from build123d import *

# Parameters (mm, degrees)
BOSS_EXTRUDE1_DEPTH = 6.35
BOSS_EXTRUDE2_DEPTH = 6.35
FILLET1_R           = 10
FILLET2_R           = 5
CUT_EXTRUDE1_DEPTH  = 7.35
SKETCH4_R           = 1.85
CUT_EXTRUDE2_DEPTH  = 7.35


with BuildPart() as part:
    # Sketch1 → Boss-Extrude1 (new body)
    with BuildSketch(Plane.XY):
        Polygon((-100, 0), (0, -100), (25.4, -100), (25.4, 25.4), (-100, 25.4), align=None)
    extrude(amount=BOSS_EXTRUDE1_DEPTH)

    # Sketch2 → Boss-Extrude2 (add)
    with BuildSketch(Plane.XY):
        Polygon((24.2, 37.7), (84.2, 37.7), (84.2, -22.3), (25.4, -100), (24.2, -22.3), (-100, 25.4), align=None)
    extrude(amount=BOSS_EXTRUDE2_DEPTH)

    # Fillet1
    fillet1_edges = [part.edges().sort_by_distance(p)[0] for p in [
        (84.2, 37.7, 3.175),
    ]]
    fillet(fillet1_edges, radius=FILLET1_R)

    # Fillet2
    fillet2_edges = [part.edges().sort_by_distance(p)[0] for p in [
        (84.2, -22.3, 3.175),
        (25.4, -100, 3.175),
        (0, -100, 3.175),
        (-100, 0, 3.175),
        (-100, 25.4, 3.175),
    ]]
    fillet(fillet2_edges, radius=FILLET2_R)

    # Sketch3 → Cut-Extrude1 (cut, through all)
    with BuildSketch(Plane.XY.offset(6.35)):
        with BuildLine():
            Line((43.7, 31.2), (64.7, 31.2))
            ThreePointArc((64.7, 31.2), (73.892388155, 27.392388155), (77.7, 18.2))
            Line((77.7, 18.2), (77.7, -2.8))
            ThreePointArc((77.7, -2.8), (73.892388155, -11.992388155), (64.7, -15.8))
            Line((64.7, -15.8), (43.7, -15.8))
            ThreePointArc((43.7, -15.8), (34.507611845, -11.992388155), (30.7, -2.8))
            Line((30.7, -2.8), (30.7, 18.2))
            ThreePointArc((30.7, 18.2), (34.507611845, 27.392388155), (43.7, 31.2))
        make_face()
    extrude(amount=-CUT_EXTRUDE1_DEPTH, mode=Mode.SUBTRACT)

    # Sketch4 → Cut-Extrude2 (cut, through all)
    with BuildSketch(Plane(origin=(0, 0, 0), x_dir=(-1, 0, 0), z_dir=(0, 0, -1))):
        with Locations((-77.581727984, 31.081727984)):
            Circle(SKETCH4_R)
        with Locations((-30.821727984, 31.081727984)):
            Circle(SKETCH4_R)
        with Locations((-30.821727984, -15.678272016)):
            Circle(SKETCH4_R)
        with Locations((-77.581727984, -15.678272016)):
            Circle(SKETCH4_R)
    extrude(amount=-CUT_EXTRUDE2_DEPTH, mode=Mode.SUBTRACT)


solid = part.part
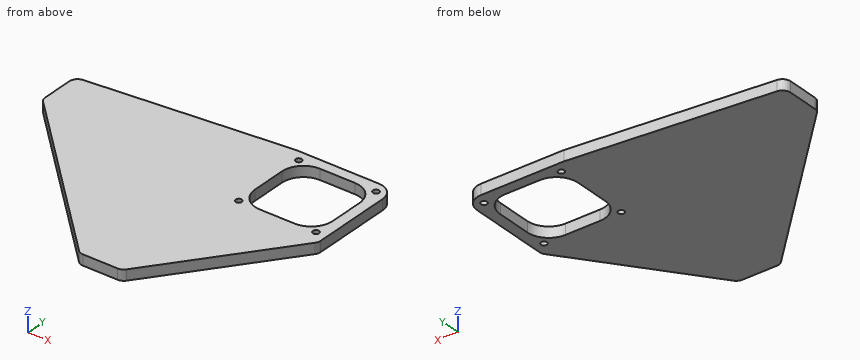
For this review, take the finished solid that the model builds, in its own axes (mm). Give positions to 0.01 mm unless a question says otherwise; leave off trailing zeros. Loops run counter-clockwise (first coordinate to the right, second up) from the corner with the lowest first, then second, coordinate; pieces in that order, holes last.
Item 1: Insertion check: pin 1 (3 mm diameter, centred on x = 49, z = 2, fed in from -Y); pin 2 (2 mm diameter, centred on x = 30.82, y = -15.68, fed in from +Z); pin 3 (2 mm diameter, centred on x = -37, z = 3, fed in from -Y). Each pin has a flat end and moves straight along its axis. Give the tip position at first contact, or say it passes through.
Item 2: Take a section at D-D, the plane x = -63. State the section outline as (y, z) points, and give its area (3 significant figures).
Item 3: Take a section at C-C, the plane y = -60.5. State the section outline as (x, z) points.
Item 4: Take a section at B-B, the plane z = 4.25. State the section outline as (x, y) points, and give its area (3 significant figures).
Item 5: For line 1 along X through (y, z) = (-10, 1); line 2 along Y through (x, z) = (65.5, 4.25); line 3 along X through (y, z) = (19.5, 5.25), list the stretches that pass through material, from the lowest coordinate up.
Item 6: Take a section at A-A, the plane x = 55. State the section outline as (y, z) points, and give its area (3 significant figures).
Calculated:
1. pin 1: stops at y = -70.8
1. pin 2: passes through
1. pin 3: stops at y = -64
2. outline: (-37, 0) - (29.06, 0) - (29.06, 6.35) - (-37, 6.35) - close
2. area: 420 mm2
3. outline: (-39.5, 0) - (55.29, 0) - (55.29, 6.35) - (-39.5, 6.35) - close
4. outline: (-100, 2.07) arc R5 ccw to (-98.54, -1.46) - (-1.46, -98.54) arc R5 ccw to (2.07, -100) - (22.91, -100) arc R5 ccw to (26.9, -98.02) - (83.19, -23.64) arc R5 ccw to (84.2, -20.62) - (84.2, 27.7) arc R10 ccw to (74.2, 37.7) - (24.2, 37.7) - (-95.49, 25.85) arc R5 ccw to (-100, 20.87) - close; hole circle Ø3.7 at (30.82, -15.68); hole circle Ø3.7 at (30.82, 31.08); hole (30.7, -2.8) arc R13 ccw to (43.7, -15.8) - (64.7, -15.8) arc R13 ccw to (77.7, -2.8) - (77.7, 18.2) arc R13 ccw to (64.7, 31.2) - (43.7, 31.2) arc R13 ccw to (30.7, 18.2) - close; hole circle Ø3.7 at (77.58, -15.68); hole circle Ø3.7 at (77.58, 31.08)
4. area: 15,200 mm2
5. line 1: x = -90 to 32.88, 75.52 to 84.2
5. line 2: y = -47.01 to -15.78, 31.18 to 37.7
5. line 3: x = -100 to 30.77, 77.63 to 84.2
6. outline: (-60.89, 0) - (-15.8, 0) - (-15.8, 6.35) - (-60.89, 6.35) - close; (31.2, 0) - (37.7, 0) - (37.7, 6.35) - (31.2, 6.35) - close
6. area: 328 mm2
